Input: dimensioned drawing with shaded views. Units: mm. Origin: part minimum x, y, z. Coordinates: 2 decimals unless noted, no trailing zeros. Loops run counter-clockwise (first coordinate to the right, second up) from the corner with the lowest first, then second, coordinate; pieces in that order, holes last. Notation, with made-up numbers: (17, 48.25) - (63, 48.25) arc R23 cw to (63, 76.25) - close; hole circle Ø2 at (3.5, -20). An arc over 180 degrees is marked (long way). Use one line per item in the form item = value. Start each with the question number.
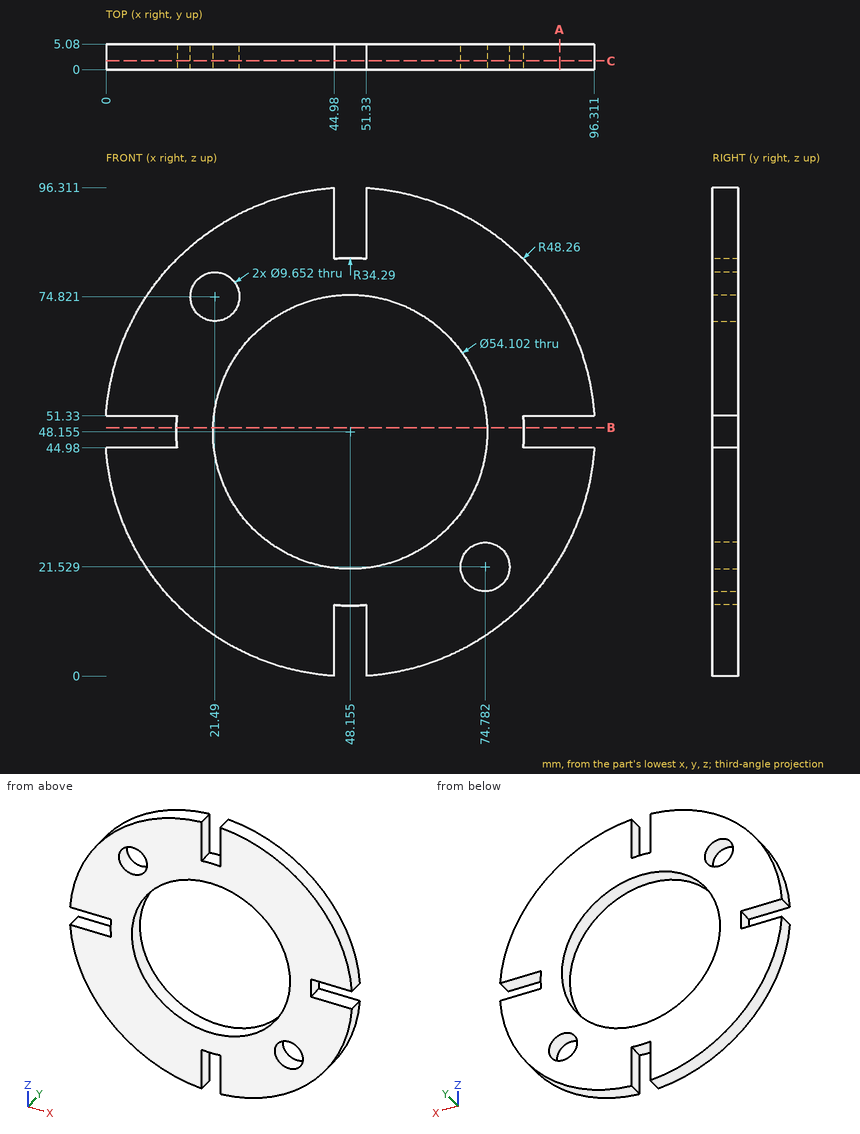
(1) Cut plane C-C, the plane y = 1.75. Output: boundary loops of the cut face in (x, z) (1 decimal).
(2) Cut plane B-B, the plane z = 49. Output: boundary loops of the cut face in (x, y) (1 decimal).
(3) Contact query for flat-ended pins moving along their axis: pin 1 (2.5 mm diameter, centred on y = 1.5, z = 9, fed in from +X) (1 decimal); pin 2 (2 mm diameter, centred on x = 42, z = 23.5, fed in from +Y); pin 3 (1.5 mm diameter, centred on y = 3, z = 8.5, fed in from -X). Output: stop coordinate, or through.
(4) Cut plane A-A, the plane x = 89.5. Output: boundary loops of the cut face in (y, z).
(5) Material intervals for line 1 (X direction, y = 2, z = 49) (1 decimal); line 2 (Z direction, x = 51, y = 2.75) (1 decimal); line 3 (X direction, y = 1.25, z = 44) (1 decimal), sorted ascending.
Recorded:
q1.outline = (0, 45) arc R48.3 ccw to (45, 0) - (45, 14) arc R34.3 ccw to (51.3, 14) - (51.3, 0) arc R48.3 ccw to (96.3, 45) - (82.3, 45) arc R34.3 ccw to (82.3, 51.3) - (96.3, 51.3) arc R48.3 ccw to (51.3, 96.3) - (51.3, 82.3) arc R34.3 ccw to (45, 82.3) - (45, 96.3) arc R48.3 ccw to (0, 51.3) - (14, 51.3) arc R34.3 ccw to (14, 45) - close; hole circle Ø9.7 at (21.5, 74.8); hole circle Ø54.1 at (48.2, 48.2); hole circle Ø9.7 at (74.8, 21.5)
q2.outline = (13.9, 0) - (21.1, 0) - (21.1, 5.1) - (13.9, 5.1) - close; (75.2, 0) - (82.4, 0) - (82.4, 5.1) - (75.2, 5.1) - close
q3.pin_1 = 78
q3.pin_2 = through
q3.pin_3 = 19.6
q4.outline = (0, 23.26) - (5.08, 23.26) - (5.08, 44.98) - (0, 44.98) - close; (0, 51.33) - (5.08, 51.33) - (5.08, 73.05) - (0, 73.05) - close
q5.line_1 = 13.9 to 21.1, 75.2 to 82.4
q5.line_2 = 14 to 21.3, 75.1 to 82.3
q5.line_3 = 0.1 to 21.4, 74.9 to 96.2
